```python
from build123d import *

# Parameters (mm, degrees)
SALIENTE_EXTRUIR1_DEPTH = 5
CROQUIS2_W              = 20
CROQUIS2_H              = 10
SALIENTE_EXTRUIR2_DEPTH = 5
CROQUIS3_R              = 5
CROQUIS3_R_2            = 1
SALIENTE_EXTRUIR4_DEPTH = 5
CROQUIS5_R              = 1
CORTAR_EXTRUIR1_DEPTH   = 5
CROQUIS7_R              = 1
CORTAR_EXTRUIR2_DEPTH   = 5


with BuildPart() as part:
    # Croquis1 → Saliente-Extruir1 (new body)
    with BuildSketch(Plane.XY):
        Polygon((10, -25), (-10, -25), (-5, 35), (5, 35), align=None)
    extrude(amount=SALIENTE_EXTRUIR1_DEPTH)

    # Croquis2 → Saliente-Extruir2 (add)
    with BuildSketch(Plane(origin=(0, -25, 0), x_dir=(-1, 0, 0), z_dir=(0, -1, 0))):
        Rectangle(CROQUIS2_W, CROQUIS2_H)
    extrude(amount=-SALIENTE_EXTRUIR2_DEPTH)

    # Croquis3 → Saliente-Extruir4 (add)
    with BuildSketch(Plane.XY.offset(5)):
        with Locations((0, 35)):
            Circle(CROQUIS3_R)
        with Locations((0, 35)):
            Circle(CROQUIS3_R_2, mode=Mode.SUBTRACT)
    extrude(amount=-SALIENTE_EXTRUIR4_DEPTH)

    # Croquis5 → Cortar-Extruir1 (cut)
    with BuildSketch(Plane.XY.offset(5)):
        with Locations((0, 35)):
            Circle(CROQUIS5_R)
    extrude(amount=-CORTAR_EXTRUIR1_DEPTH, mode=Mode.SUBTRACT)

    # Croquis7 → Cortar-Extruir2 (cut)
    with BuildSketch(Plane.XZ.offset(25)):
        with Locations(Location((0, 0, 0), (0, 0, 270))):
            Circle(CROQUIS7_R)
    extrude(amount=-CORTAR_EXTRUIR2_DEPTH, mode=Mode.SUBTRACT)


solid = part.part
```
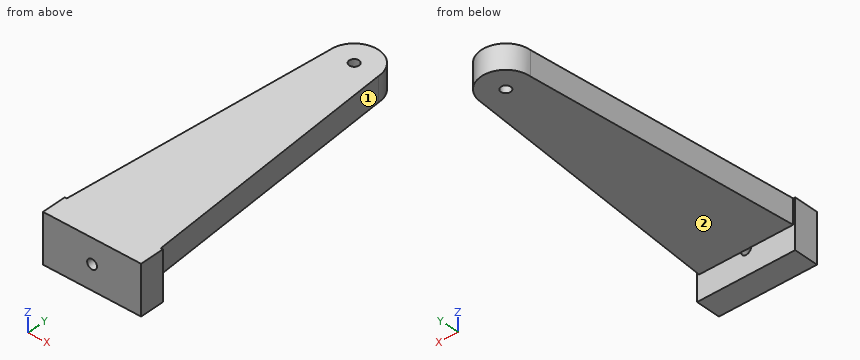
For this review, take the finished solid that the model builds, in its own axes (mm). Face numbers are marked on the shaded views. A direction names the side the tool comes from. Give positions to 0.01 mm unless a question says otherwise; leave off trailing zeros. Write each loop counter-clockwise with the first axis right and the second up, starting at its lowest first coordinate (ties: lowest second). Pieces come first, ordered by that corner, then holes.
Item 1: Insertion check: P1, Ø3, axis at y = -3.5, z = 3.5, coming from the -X side; P2, Ø6, axis at x = 3, y = -4.5, coming from the -Z side; P3, Ø1, axis at x = 2.5, z = 0, coming from the +Y side. Each pin has a flat end and moves straight along its axis. Give the tip position at first contact, or say it passes through.
Item 2: Take a section at D-D (y = 23). Give the boundary of the cut face in (x, z).
Item 3: Take a section at C-C (x = -5.75). Give the boundary of the cut face in (y, z), and give its area (3 significant figures).
Item 4: Machinability: for the marked faces 1 and 2, which of the approach directions +Z, -Z, +X, -X, +Y, -Y give a long, thin tool a straight path to every point of the face, cutting with its end or side? Answer none if there is none.
Item 5: Take a section at B-B (z = 3.5). Give the boundary of the cut face in (x, y).
Item 6: Take a section at A-A (x = 0). Give the boundary of the cut face in (y, z).
Item 7: Wall thickness on probe 1 along Y at (x, z) = (0, 4); probe 2 along X at (y, z) = (-23.2, 0); probe 3 along Z at (x, y) = (5.5, -1.5): over which ranges is each line inside the solid? List them lowest first.
Established:
1. P1: stops at x = -8.33
1. P2: stops at z = 0
1. P3: stops at y = 39.58
2. outline: (-6, 0) - (6, 0) - (6, 5) - (-6, 5) - close
3. outline: (-25, -5) - (-20, -5) - (-20, 0) - (26, 0) - (26, 5) - (-25, 5) - close
3. area: 280 mm2
4. face 1: +Z, -Z, +X, +Y
4. face 2: -Z, +X, -X, +Y
5. outline: (-10, -25) - (10, -25) - (10, -20) - (9.58, -20) - (5, 35) arc R5 ccw to (-5, 35) - (-9.58, -20) - (-10, -20) - close; hole circle Ø2 at (0, 35)
6. outline: (-25, -5) - (-20, -5) - (-20, -1) - (-25, -1) - close; (-25, 1) - (-20, 1) - (-20, 0) - (34, 0) - (34, 5) - (-25, 5) - close; (36, 0) - (40, 0) - (40, 5) - (36, 5) - close
7. probe 1: y = -25 to 34, 36 to 40
7. probe 2: x = -10 to -1, 1 to 10
7. probe 3: z = 0 to 5
